```python
from build123d import *

# Parameters (mm, degrees)
SKETCH1_W           = 162
SKETCH1_H           = 162
SKETCH1_W_2         = 50
SKETCH1_H_2         = 50
BOSS_EXTRUDE1_DEPTH = 23
SKETCH1_2_W         = 162
SKETCH1_2_H         = 162
SKETCH1_2_W_2       = 50
SKETCH1_2_H_2       = 50
BOSS_EXTRUDE2_DEPTH = 3


with BuildPart() as part:
    # Sketch1 → Boss-Extrude1 (new body)
    with BuildSketch(Plane.XY):
        with Locations((2.220930233, -28.593023256)):
            Rectangle(SKETCH1_W, SKETCH1_H)
        with Locations((-50.779069767, 24.406976744)):
            Rectangle(SKETCH1_W_2, SKETCH1_H_2, mode=Mode.SUBTRACT)
        with Locations((2.220930233, 24.406976744)):
            Rectangle(SKETCH1_W_2, SKETCH1_H_2, mode=Mode.SUBTRACT)
        with Locations((55.220930233, 24.406976744)):
            Rectangle(SKETCH1_W_2, SKETCH1_H_2, mode=Mode.SUBTRACT)
        with Locations((-50.779069767, -28.593023256)):
            Rectangle(SKETCH1_W_2, SKETCH1_H_2, mode=Mode.SUBTRACT)
        with Locations((2.220930233, -28.593023256)):
            Rectangle(SKETCH1_W_2, SKETCH1_H_2, mode=Mode.SUBTRACT)
        with Locations((55.220930233, -28.593023256)):
            Rectangle(SKETCH1_W_2, SKETCH1_H_2, mode=Mode.SUBTRACT)
        with Locations((-50.779069767, -81.593023256)):
            Rectangle(SKETCH1_W_2, SKETCH1_H_2, mode=Mode.SUBTRACT)
        with Locations((2.220930233, -81.593023256)):
            Rectangle(SKETCH1_W_2, SKETCH1_H_2, mode=Mode.SUBTRACT)
        with Locations((55.220930233, -81.593023256)):
            Rectangle(SKETCH1_W_2, SKETCH1_H_2, mode=Mode.SUBTRACT)
    extrude(amount=BOSS_EXTRUDE1_DEPTH)

    # Sketch1_2 → Boss-Extrude2 (add)
    # profile 1 of 10: a face of its own
    with BuildSketch(Plane.XY):
        with Locations((2.220930233, -28.593023256)):
            Rectangle(SKETCH1_2_W, SKETCH1_2_H)
        with Locations((-50.779069767, 24.406976744)):
            Rectangle(SKETCH1_2_W_2, SKETCH1_2_H_2, mode=Mode.SUBTRACT)
        with Locations((2.220930233, 24.406976744)):
            Rectangle(SKETCH1_2_W_2, SKETCH1_2_H_2, mode=Mode.SUBTRACT)
        with Locations((55.220930233, 24.406976744)):
            Rectangle(SKETCH1_2_W_2, SKETCH1_2_H_2, mode=Mode.SUBTRACT)
        with Locations((-50.779069767, -28.593023256)):
            Rectangle(SKETCH1_2_W_2, SKETCH1_2_H_2, mode=Mode.SUBTRACT)
        with Locations((2.220930233, -28.593023256)):
            Rectangle(SKETCH1_2_W_2, SKETCH1_2_H_2, mode=Mode.SUBTRACT)
        with Locations((55.220930233, -28.593023256)):
            Rectangle(SKETCH1_2_W_2, SKETCH1_2_H_2, mode=Mode.SUBTRACT)
        with Locations((-50.779069767, -81.593023256)):
            Rectangle(SKETCH1_2_W_2, SKETCH1_2_H_2, mode=Mode.SUBTRACT)
        with Locations((2.220930233, -81.593023256)):
            Rectangle(SKETCH1_2_W_2, SKETCH1_2_H_2, mode=Mode.SUBTRACT)
        with Locations((55.220930233, -81.593023256)):
            Rectangle(SKETCH1_2_W_2, SKETCH1_2_H_2, mode=Mode.SUBTRACT)
    # profile 2 of 10: a face of its own
    with BuildSketch(Plane.XY):
        with Locations((55.220930233, -81.593023256)):
            Rectangle(SKETCH1_2_W_2, SKETCH1_2_H_2)
    # profile 3 of 10: a face of its own
    with BuildSketch(Plane.XY):
        with Locations((2.220930233, -81.593023256)):
            Rectangle(SKETCH1_2_W_2, SKETCH1_2_H_2)
    # profile 4 of 10: a face of its own
    with BuildSketch(Plane.XY):
        with Locations((-50.779069767, -81.593023256)):
            Rectangle(SKETCH1_2_W_2, SKETCH1_2_H_2)
    # profile 5 of 10: a face of its own
    with BuildSketch(Plane.XY):
        with Locations((-50.779069767, -28.593023256)):
            Rectangle(SKETCH1_2_W_2, SKETCH1_2_H_2)
    # profile 6 of 10: a face of its own
    with BuildSketch(Plane.XY):
        with Locations((2.220930233, -28.593023256)):
            Rectangle(SKETCH1_2_W_2, SKETCH1_2_H_2)
    # profile 7 of 10: a face of its own
    with BuildSketch(Plane.XY):
        with Locations((55.220930233, -28.593023256)):
            Rectangle(SKETCH1_2_W_2, SKETCH1_2_H_2)
    # profile 8 of 10: a face of its own
    with BuildSketch(Plane.XY):
        with Locations((55.220930233, 24.406976744)):
            Rectangle(SKETCH1_2_W_2, SKETCH1_2_H_2)
    # profile 9 of 10: a face of its own
    with BuildSketch(Plane.XY):
        with Locations((2.220930233, 24.406976744)):
            Rectangle(SKETCH1_2_W_2, SKETCH1_2_H_2)
    # profile 10 of 10: a face of its own
    with BuildSketch(Plane.XY):
        with Locations((-50.779069767, 24.406976744)):
            Rectangle(SKETCH1_2_W_2, SKETCH1_2_H_2)
    extrude(amount=BOSS_EXTRUDE2_DEPTH)


solid = part.part
```
Can you work these out from the model? Positions are in its coordinate system, mm. Give positions to 0.01 mm unless a question says otherwise; leave off trailing zeros. Loops run counter-clockwise (first coordinate to the right, second up) from the corner with the lowest first, then second, coordinate; pieces in that order, holes last. Notation, with made-up numbers: M 53,84 L 94,84 A35 cw 94,121 Z; hole C 44,59.5 d11. An arc over 180 degrees is marked long. One line per item, written item: value.
(1) Suppose I cut it at B-B on y = -5.5. List the corners of the cut face in (x, z) for me, plus the area to 3 significant figures.
Returned:
outline: M -78.78,0 L 83.22,0 L 83.22,23 L 80.22,23 L 80.22,3 L 30.22,3 L 30.22,23 L 27.22,23 L 27.22,3 L -22.78,3 L -22.78,23 L -25.78,23 L -25.78,3 L -75.78,3 L -75.78,23 L -78.78,23 Z
area: 726 mm^2
(2) Will this pin go through, and if not, where does the flat tip stop? pin 1 (2 mm diameter, centred on x = 53, y = -84.5, fed in from +Z).
Returned:
pin 1: z = 3
(3) We'd pull the mould along Y, two halves only. Please class faces 1 (the face through (83.221, -30, 11)), 2 (the face through (-51, 49.407, 13)): released by +Y, released by -Y, zero draft, split by the parting line, or undercut.
Returned:
face 1: zero draft
face 2: undercut
(4) Suppose I cut it at C-C on z = 21. Count the separate pieces of the cut face and the enclosed holes in it, plus the area to 3 significant figures.
Returned:
separate pieces: 1
enclosed holes: 9
area: 3,740 mm^2
(5) Suppose I cut it at A-A on x = 22.5. List the corners of the cut face in (y, z) for me.
Returned:
outline: M -109.59,0 L 52.41,0 L 52.41,23 L 49.41,23 L 49.41,3 L -0.59,3 L -0.59,23 L -3.59,23 L -3.59,3 L -53.59,3 L -53.59,23 L -56.59,23 L -56.59,3 L -106.59,3 L -106.59,23 L -109.59,23 Z
(6) I need wall thicknesses on line 1 (X direction, y = -25, z = 11); line 2 (Y direction, x = 63.5, z = 15); line 3 (Z direction, x = 33, y = -46). Which ranges of each line are inside material? Lowest first, please.
Returned:
line 1: -78.78 to -75.78, -25.78 to -22.78, 27.22 to 30.22, 80.22 to 83.22
line 2: -109.59 to -106.59, -56.59 to -53.59, -3.59 to -0.59, 49.41 to 52.41
line 3: 0 to 3
